from build123d import *

# Parameters (mm, degrees)
SKETCH1_W           = 20
SKETCH1_H           = 2.5
BOSS_EXTRUDE1_DEPTH = 28
SKETCH7_W           = 1.25
SKETCH7_H           = 5
BOSS_EXTRUDE3_DEPTH = 5
FILLET1_R           = 2.5
SKETCH8_R           = 0.75
CUT_EXTRUDE3_DEPTH  = 38.569302663
CHAMFER1_SIZE       = 1


with BuildPart() as part:
    # Sketch1 → Boss-Extrude1 (new body)
    with BuildSketch(Plane.XY):
        Rectangle(SKETCH1_W, SKETCH1_H)
    extrude(amount=BOSS_EXTRUDE1_DEPTH)

    # Sketch3 → section 0 of loft1
    with BuildSketch(Plane.XY.offset(31), mode=Mode.PRIVATE) as loft1_s0:
        with BuildLine():
            Line((-4.55, 2.5), (0.45, 2.5))
            Line((0.45, 2.5), (0.45, -2.5))
            Line((0.45, -2.5), (-4.55, -2.5))
            Line((-4.55, -2.5), (-4.55, 2.5))
        make_face()
    # loft up to a face of the part (loft1)
    loft([loft1_s0.sketch, part.faces().sort_by_distance((0, 0, 28))[0]])

    # Sketch7 → Boss-Extrude3 (add)
    with BuildSketch(Plane.XY.offset(31)):
        with Locations((-3.925, 0)):
            Rectangle(SKETCH7_W, SKETCH7_H)
        with Locations((-0.175, 0)):
            Rectangle(SKETCH7_W, SKETCH7_H)
    extrude(amount=BOSS_EXTRUDE3_DEPTH)

    # Fillet1
    fillet1_edges = [part.edges().sort_by_distance(p)[0] for p in [
        (-0.175, -2.5, 36),
        (-3.925, -2.5, 36),
        (-3.925, 2.5, 36),
        (-0.175, 2.5, 36),
    ]]
    fillet(fillet1_edges, radius=FILLET1_R - 0.0001)  # a hair under: the kernel refuses the full size

    # Sketch8 → Cut-Extrude3 (cut, through all)
    with BuildSketch(Plane(origin=(0.45, 0, 0), x_dir=(0, 0, -1), z_dir=(1, 0, 0))):
        with Locations((-33.5, 0)):
            Circle(SKETCH8_R)
    extrude(amount=-CUT_EXTRUDE3_DEPTH, mode=Mode.SUBTRACT)

    # Chamfer1
    chamfer1_edges = [part.edges().sort_by_distance(p)[0] for p in [
        (0, -1.25, 0),
        (-10, 0, 0),
        (0, 1.25, 0),
        (10, 0, 0),
    ]]
    chamfer(chamfer1_edges, length=CHAMFER1_SIZE)


solid = part.part
Work out the finished part from the listing and answer in its coordinate system (mm). A direction names the side the tool comes from. Give positions to 0.01 mm unless a question says otherwise; leave off trailing zeros. Order: outer loops, then holes, each group sorted by start corner. A loop starts at its lowest first (then second) coordinate and runs counter-clockwise, first axis right, second up. Notation, with made-up numbers: (-14, -25) -> (36, -25) arc R27 cw to (36, -5) -> close; hole circle Ø10 at (-7, 71). An arc over 180 degrees is marked (long way). Answer as a JSON object with one key per item and string values. Group by question number.
1. The mould has two halves that part along Y. Classify faces 1 (the cylindrical face through (0, 2, 35)), 2 (the flat face through (-4.55, 1, 33)), 3 (the cylindrical face through (-3.916, 0.225, 32.785)): released by +Y, released by -Y, zero draft, split by the parting line, or undercut.
2. Section A-A on z = 19.5 is taken. Determine the outline of the cut face in (x, y).
3. Flat-ended cylindrical pins translate along their axes: pin 1 Ø1 at (x, y) = (-7.5, -0.5) entering from +Z; pin 2 Ø3 at (x, z) = (-2.5, 13.5) entering from +Y; pin 3 Ø1.5 at (y, z) = (-1, 34) entering from -X. Find the tip coordinate at first contact, or state that the pin passes through.
4. Consider line 1 along Y through (x, z) = (-0.25, 33.5); line 2 along X through (y, z) = (-0.8, 32); line 3 along Y through (x, z) = (8.25, 27). Determine where each line is inside the solid, lowest interval first. Write a range as [from, to].
5. A tool of negligible diameter and unlimited length cuts with its end or side. For faces 4 (the flat face through (0, -1.25, 14)), 5 (the flat face through (-0.8, 1, 33)), 6 (the flat face through (0, 1.25, 14)), 7 (the cylindrical face through (-0.166, 0.225, 32.785)), 8 (the cylindrical face through (-4, -2, 35)), from which of +Z, -Z, +X, -X, +Y, -Y can it reach the whole face along a straight path? Write none if from no direction.
Result sheet:
{
 "1": {"face 1": "released by +Y", "face 2": "zero draft", "face 3": "undercut"},
 "2": {"outline": "(-10, -1.25) -> (10, -1.25) -> (10, 1.25) -> (-10, 1.25) -> close"},
 "3": {"pin 1": "stops at z = 29.65", "pin 2": "stops at y = 1.25", "pin 3": "stops at x = -4.55"},
 "4": {"line 1": "y = [-2.5, -0.75], [0.75, 2.5]", "line 2": "x = [-4.55, -3.3], [-0.8, 0.45]", "line 3": "y = [-1.25, 1.25]"},
 "5": {"face 4": "-Z, +X, -X, -Y", "face 5": "+Z, +Y, -Y", "face 6": "-Z, +X, -X, +Y", "face 7": "+X, -X", "face 8": "+Z, +X, -X, -Y"}
}
